Geometry: final body of the model. Coordinates: model frame, mm. Face numbers are marked on the shaded views. A direction names the side the tool comes from. Give positions to 0.01 mm unless a question says otherwise; leave off trailing zeros. Order: outer loops, then holes, each group sorted by start corner. A loop starts at its lowest first (then second) coordinate and runs counter-clockwise, first axis right, second up. Notation, with made-up numbers: (-13.5, 37) - (28.5, 37) arc R32 cw to (28.5, 65) - close; hole circle Ø1 at (83.5, -3). An arc over 180 degrees is marked (long way). Use one line per item in the form item = value.
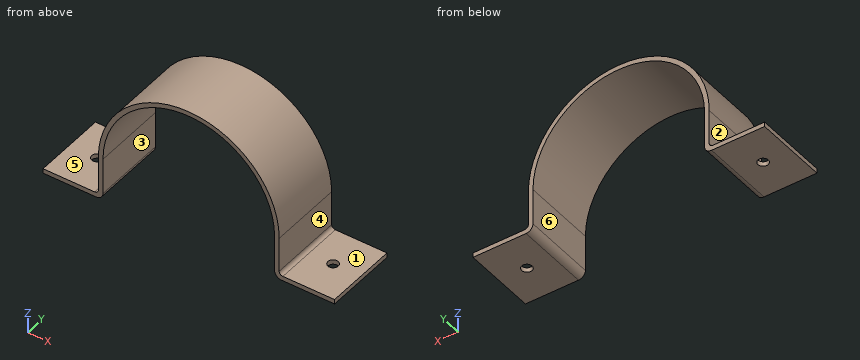
from build123d import *

# Parameters (mm, degrees)
F1_DEPTH = 50.8
F3_R     = 9.525
F4_R     = 5.08
F2_R     = 7.14375
F5_DEPTH = 25.4


with BuildPart() as f1:
    # F0 (on Front) → F1 (new body, symmetric)
    with BuildSketch(Plane.XZ):
        with BuildLine():
            ThreePointArc((-118.11, 0), (0, 118.11), (118.11, 0))
            Line((118.11, 0), (118.11, -59.055))
            Line((118.11, -59.055), (200.66, -59.055))
            Line((200.66, -59.055), (200.66, -52.705))
            Line((200.66, -52.705), (124.46, -52.705))
            Line((124.46, -52.705), (124.46, 0))
            ThreePointArc((124.46, 0), (0, 124.46), (-124.46, 0))
            Line((-124.46, 0), (-124.46, -52.705))
            Line((-124.46, -52.705), (-200.66, -52.705))
            Line((-200.66, -52.705), (-200.66, -59.055))
            Line((-200.66, -59.055), (-118.11, -59.055))
            Line((-118.11, -59.055), (-118.11, 0))
        make_face()
    extrude(amount=F1_DEPTH, both=True)

    # F3
    f3_edges = [f1.edges().sort_by_distance(p)[0] for p in [
        (-118.11, 0, -59.055),
        (118.11, 0, -59.055),
    ]]
    fillet(f3_edges, radius=F3_R)

    # F4
    f4_edges = [f1.edges().sort_by_distance(p)[0] for p in [
        (-124.46, 0, -52.705),
        (124.46, 0, -52.705),
    ]]
    fillet(f4_edges, radius=F4_R)

    # F2 (on face) → F5 (cut)
    with BuildSketch(Plane(origin=(0, 0, -59.055), x_dir=(1, 0, 0), z_dir=(0, 0, -1))):
        with Locations((-162.56, 0)):
            Circle(F2_R)
        with Locations((162.56, 0)):
            Circle(F2_R)
    extrude(amount=-F5_DEPTH, mode=Mode.SUBTRACT)


solid = f1.part
(1) Cut plane A-A on y = 0. Output: boundary loops of the cut face in (x, z) (3 decimals), plus the area to 3 significant figures.
Computed values:
outline = (-200.66, -59.055) - (-169.704, -59.055) - (-169.704, -52.705) - (-200.66, -52.705) - close; (-155.416, -59.055) - (-127.635, -59.055) arc R9.525 ccw to (-118.11, -49.53) - (-118.11, 0) arc R118.11 cw to (118.11, 0) - (118.11, -49.53) arc R9.525 ccw to (127.635, -59.055) - (155.416, -59.055) - (155.416, -52.705) - (129.54, -52.705) arc R5.08 cw to (124.46, -47.625) - (124.46, 0) arc R124.46 ccw to (-124.46, 0) - (-124.46, -47.625) arc R5.08 cw to (-129.54, -52.705) - (-155.416, -52.705) - close; (169.704, -59.055) - (200.66, -59.055) - (200.66, -52.705) - (169.704, -52.705) - close
area = 3,930 mm²
(2) Cut plane C-C on z = -32. Output: boundary loops of the cut face in (x, y), plus the area to 3 significant figures.
Computed values:
outline = (-124.46, -50.8) - (-118.11, -50.8) - (-118.11, 50.8) - (-124.46, 50.8) - close; (118.11, -50.8) - (124.46, -50.8) - (124.46, 50.8) - (118.11, 50.8) - close
area = 1,290 mm²
(3) Cut plane B-B on x = 162.56. Output: boundary loops of the cut face in (y, z) (3 decimals), plus the area to 3 significant figures.
Computed values:
outline = (-50.8, -59.055) - (-7.144, -59.055) - (-7.144, -52.705) - (-50.8, -52.705) - close; (7.144, -59.055) - (50.8, -59.055) - (50.8, -52.705) - (7.144, -52.705) - close
area = 554 mm²
(4) Contact query for flat-ended pins moving along their axis: pin 1 Ø3 at (x, y) = (-124.5, -21) entering from -Z; pin 2 Ø15 at (y, z) = (2.5, -19.5) entering from -X; pin 3 Ø12 at (y, z) = (-27.5, 97.5) entering from -X. Output: stop coordinate, or through.
Computed values:
pin_1 = -58.91
pin_2 = -124.46
pin_3 = -84.37
(5) Cut plane D-D on y = 25.5. Output: boundary loops of the cut face in (x, z) (3 decimals), plus the area to 3 significant figures.
Computed values:
outline = (-200.66, -59.055) - (-127.635, -59.055) arc R9.525 ccw to (-118.11, -49.53) - (-118.11, 0) arc R118.11 cw to (118.11, 0) - (118.11, -49.53) arc R9.525 ccw to (127.635, -59.055) - (200.66, -59.055) - (200.66, -52.705) - (129.54, -52.705) arc R5.08 cw to (124.46, -47.625) - (124.46, 0) arc R124.46 ccw to (-124.46, 0) - (-124.46, -47.625) arc R5.08 cw to (-129.54, -52.705) - (-200.66, -52.705) - close
area = 4,110 mm²
(6) Reachability of the marked faces 1, 2 and 3 from +Z, -Z, +X, -X, +Y, -Y: full face, straight path, thin tool, end or side. Return the list, or none.
Computed values:
face_1 = +Z, +X, +Y, -Y
face_2 = +Z, -X, +Y, -Y
face_3 = -Z, +Y, -Y
(7) Ray query, line 1 along Y through (x, z) = (162, -57); line 2 along X through (y, z) = (-20, -36); line 3 along X through (y, z) = (0, -56.5). Return the intervals inside material, ascending.
Computed values:
line_1 = -50.8 to -7.12, 7.12 to 50.8
line_2 = -124.46 to -118.11, 118.11 to 124.46
line_3 = -200.66 to -169.7, -155.42 to -121.14, 121.14 to 155.42, 169.7 to 200.66
(8) Pull-direction query (X, two-part tool) for the marked faces 4, 5 and 6; classes: released by +X, released by -X, zero draft, split by the parting line, or undercut.
Computed values:
face_4 = released by +X
face_5 = zero draft
face_6 = undercut
